Geometry check sheet. Reference: the model listing, model coordinates, mm. Face numbers are marked on the shaded views. Coordinates: 2 decimals unless noted, no trailing zeros. Loops run counter-clockwise (first coordinate to the right, second up) from the corner with the lowest first, then second, coordinate; pieces in that order, holes last. Notation, with made-up numbers: (51, -6) - (86, -6) arc R30 cw to (86, 33) - close; hole circle Ø4 at (-32.75, 45). An arc over 180 degrees is marked (long way). One line per item, written item: value.
from build123d import *

# Parameters (mm, degrees)
SKIZZE1_R                       = 23.5
AUFSATZ_LINEAR_AUSTRAGEN1_DEPTH = 26
F_9_0_9_DURCHMESSER_BOHRUNG1_D  = 9
SKIZZE5_W                       = 1.85
SKIZZE5_H                       = 1.75
SCHNITT_LINEAR_AUSTRAGEN1_DEPTH = 14
M6_GEWINDEBOHRUNG1_D            = 5
M6_GEWINDEBOHRUNG1_DEPTH        = 17
M6_GEWINDEBOHRUNG1_TIP          = 1.502151548
SCHNITT_LINEAR_AUSTRAGEN2_DEPTH = 171.434738243
M6_GEWINDEBOHRUNG2_D            = 5


with BuildPart() as part:
    # Skizze1 → Aufsatz-Linear austragen1 (new body)
    with BuildSketch(Plane.XY):
        with BuildLine():
            Line((31, 90), (16, 90))
            Line((16, 90), (16, -90))
            Line((16, -90), (31, -90))
            Line((31, -90), (36, -95))
            Line((36, -95), (36, -130))
            ThreePointArc((36, -130), (0, -166), (-36, -130))
            Line((-36, -130), (-36, 130))
            ThreePointArc((-36, 130), (0, 166), (36, 130))
            Line((36, 130), (36, 95))
            Line((36, 95), (31, 90))
        make_face()
        with Locations(Location((0, -130, 0), (0, 0, 180))):
            Circle(SKIZZE1_R, mode=Mode.SUBTRACT)
        with Locations(Location((0, 130, 0), (0, 0, 180))):
            Circle(SKIZZE1_R, mode=Mode.SUBTRACT)
    extrude(amount=AUFSATZ_LINEAR_AUSTRAGEN1_DEPTH)

    # Ø9.0 (9) Durchmesser Bohrung1 (through all)
    with Locations(Plane.XY.offset(26)):
        with Locations((-26, 50), (-26, -50)):
            Hole(F_9_0_9_DURCHMESSER_BOHRUNG1_D / 2)

    # Skizze5 → Schnitt-Rotation1 (revolve, cut)
    with BuildSketch(Plane(origin=(0, 0, 0), x_dir=(0, 0, -1), z_dir=(1, 0, 0)), mode=Mode.PRIVATE) as schnitt_rotation1_sk:
        with Locations((-20.925, 154.375)):
            Rectangle(SKIZZE5_W, SKIZZE5_H)
        with Locations((-5.075, 154.375)):
            Rectangle(SKIZZE5_W, SKIZZE5_H)
    schnitt_rotation1 = revolve(schnitt_rotation1_sk.sketch.rotate(Axis((0, 130, 39.739957874), (0, 0, -1)), 270), axis=Axis((0, 130, 39.739957874), (0, 0, -1)), mode=Mode.SUBTRACT)

    # Spiegeln1: Schnitt-Rotation1 across plane
    add(schnitt_rotation1.mirror(Plane.ZX), mode=Mode.SUBTRACT)

    # Skizze6 → Schnitt-Linear austragen1 (cut)
    with BuildSketch(Plane(origin=(0, 0, 0), x_dir=(-1, 0, 0), z_dir=(0, 0, -1))):
        with BuildLine():
            Line((-16, -40), (-16, 80))
            Line((-16, 80), (-5, 80))
            ThreePointArc((-5, 80), (9.849242405, 73.849242405), (16, 59))
            Line((16, 59), (16, -19))
            ThreePointArc((16, -19), (9.849242405, -33.849242405), (-5, -40))
            Line((-5, -40), (-16, -40))
        make_face()
    extrude(amount=-SCHNITT_LINEAR_AUSTRAGEN1_DEPTH, mode=Mode.SUBTRACT)

    # M6 Gewindebohrung1
    with Locations(Plane.ZY.offset(36)):
        with Locations((11.4, 63), (11.4, -82)):
            Hole(M6_GEWINDEBOHRUNG1_D / 2, depth=M6_GEWINDEBOHRUNG1_DEPTH)
            with Locations((0, 0, -(M6_GEWINDEBOHRUNG1_DEPTH + M6_GEWINDEBOHRUNG1_TIP / 2))):  # 118° drill point
                Cone(0, M6_GEWINDEBOHRUNG1_D / 2, M6_GEWINDEBOHRUNG1_TIP, mode=Mode.SUBTRACT)

    # Skizze9 → Schnitt-Linear austragen2 (cut, through all)
    with BuildSketch(Plane(origin=(0, 0, 14), x_dir=(-1, 0, 0), z_dir=(0, 0, -1))):
        with BuildLine():
            Line((-10, 73.5), (-16, 73.5))
            Line((-16, 73.5), (-16, 46.5))
            Line((-16, 46.5), (-10, 46.5))
            ThreePointArc((-10, 46.5), (3.5, 60), (-10, 73.5))
        make_face()
        with BuildLine():
            Line((-10, -6.5), (-16, -6.5))
            Line((-16, -6.5), (-16, -33.5))
            Line((-16, -33.5), (-10, -33.5))
            ThreePointArc((-10, -33.5), (3.5, -20), (-10, -6.5))
        make_face()
    extrude(amount=-SCHNITT_LINEAR_AUSTRAGEN2_DEPTH, mode=Mode.SUBTRACT)

    # M6 Gewindebohrung2 (through all)
    with Locations(Plane.XY.offset(26)):
        with Locations((4, 90)):
            Hole(M6_GEWINDEBOHRUNG2_D / 2)


solid = part.part
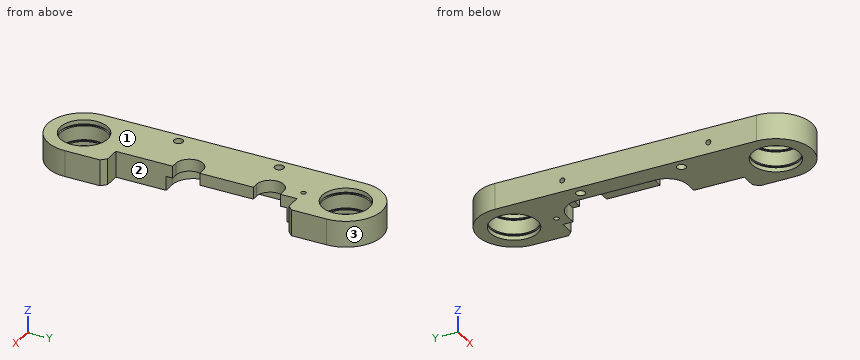
(1) Cross-section at B-B on y = 50. Record the cut outline in (x, z), and give its area (3 significant figures).
Reply:
outline: (-36, 0) - (-30.5, 0) - (-30.5, 26) - (-36, 26) - close; (-21.5, 0) - (-16, 0) - (-16, 14) - (0.93, 14) - (0.93, 26) - (-21.5, 26) - close
area: 489 mm2
(2) Go/stop test with flat-tipped pins: pin 1 Ø4 at (y, z) = (38, 8) entering from +X; pin 2 Ø1.5 at (y, z) = (87, 14) entering from +X; pin 3 Ø6 at (x, z) = (26, 13) entering from -Y. Record where each tip stops, or that it passes through.
Reply:
pin 1: x = -16
pin 2: x = 16
pin 3: y = -157.69
(3) Release check for a two-part mould opening along Y. For the marked faces 1, 2 and 3 record: pulls with the +Y half, pulls with the -Y half, needs draft (parallel to the pull), parting line crosses it, or undercut.
Reply:
face 1: needs draft
face 2: undercut
face 3: pulls with the +Y half
(4) Material ranges on probe 1 along Z at (x, y) = (-23, -82); probe 2 along Y at (x, z) = (17, 24); probe 3 along X at (y, z) = (130, 22.75), recorded low to high. Write a range as from..to.
Reply:
probe 1: 0..8.9, 13.9..26
probe 2: -161.73..-146.22, -113.78..-90, 90..113.78, 146.22..161.73
probe 3: -36..-23.5, 23.5..36
(5) Cross-section at A-A on y = -50. Record the cut outline in (x, z), and give its area (3 significant figures).
Reply:
outline: (-36, 0) - (-30.5, 0) - (-30.5, 26) - (-36, 26) - close; (-21.5, 0) - (16, 0) - (16, 26) - (-21.5, 26) - close
area: 1,120 mm2
